Read the model definition and answer for the solid it produces. Units are mm, in the model's axes. A direction names the side the tool comes from. Give positions to 0.01 mm unless a question says otherwise; leave off trailing zeros. Loops run counter-clockwise (first coordinate to the right, second up) from the corner with the lowest first, then second, coordinate; pieces in that order, holes last. Notation, with made-up numbers: (-20, 89) -> (25, 89) arc R27 ccw to (25, 121) -> close; hole circle Ø1 at (24, 13). An arc over 180 degrees is marked (long way). One line per item, written item: value. Start each with the question number.
from build123d import *

# Parameters (mm, degrees)
SKETCH1_R           = 36
BOSS_EXTRUDE1_DEPTH = 6.35
SKETCH2_R           = 29
CUT_EXTRUDE1_DEPTH  = 52.306164347
BOSS_EXTRUDE2_START = 10
SKETCH3_R           = 45
SKETCH3_R_2         = 29
BOSS_EXTRUDE2_DEPTH = 10
CUT_EXTRUDE2_DEPTH  = 10
CUT_SWEEP1_START    = -7.7
CUT_SWEEP1_DEPTH    = 7.7
CUT_SWEEP2_START    = -7.7
CUT_SWEEP2_DEPTH    = 7.7


# Read off the part's stored shape, not the designer's step: Cut-Sweep1, Cut-Sweep2
with BuildPart() as part:
    # Sketch1 → Boss-Extrude1 (new body)
    with BuildSketch(Plane(origin=(0, 0, 0), x_dir=(1, 0, 0), z_dir=(0, 1, 0))):
        with Locations(Location((0, 0, 0), (0, 0, 270))):
            Circle(SKETCH1_R)
    extrude(amount=BOSS_EXTRUDE1_DEPTH)

    # Sketch2 → Cut-Extrude1 (cut, through all)
    with BuildSketch(Plane(origin=(0, 0, 0), x_dir=(-1, 0, 0), z_dir=(0, -1, 0))):
        with Locations(Location((0, 0, 0), (0, 0, 90))):
            Circle(SKETCH2_R)
    extrude(amount=-CUT_EXTRUDE1_DEPTH, mode=Mode.SUBTRACT)

    # Sketch3 → Boss-Extrude2 (add)
    with BuildSketch(Plane.XZ.offset(BOSS_EXTRUDE2_START)):
        with Locations(Location((0, 0, 0), (0, 0, 270))):
            Circle(SKETCH3_R)
        with Locations(Location((0, 0, 0), (0, 0, 270))):
            Circle(SKETCH3_R_2, mode=Mode.SUBTRACT)
    extrude(amount=-BOSS_EXTRUDE2_DEPTH)

    # Sketch6 → Cut-Extrude2 (cut)
    with BuildSketch(Plane(origin=(0, -10, 0), x_dir=(-1, 0, 0), z_dir=(0, -1, 0))):
        with BuildLine():
            Line((9.5, -29), (9.5, -27.399817518))
            ThreePointArc((9.5, -27.399817518), (0, -29), (-9.5, -27.399817518))
            Line((-9.5, -27.399817518), (-9.5, -29))
            Line((-9.5, -29), (-9.5, -32))
            Line((-9.5, -32), (9.5, -32))
            Line((9.5, -32), (9.5, -29))
        make_face()
        with BuildLine():
            Line((9.5, 29), (9.5, 27.399817518))
            ThreePointArc((9.5, 27.399817518), (0, 29), (-9.5, 27.399817518))
            Line((-9.5, 27.399817518), (-9.5, 29))
            Line((-9.5, 29), (-9.5, 32))
            Line((-9.5, 32), (9.5, 32))
            Line((9.5, 32), (9.5, 29))
        make_face()
    extrude(amount=-CUT_EXTRUDE2_DEPTH, mode=Mode.SUBTRACT)

    # Cut-Sweep1 outline → Cut-Sweep1 (cut)
    with BuildSketch(Plane(origin=(0, 0, 0), x_dir=(1, 0, 0), z_dir=(0, 1, 0)).offset(CUT_SWEEP1_START)):
        with BuildLine():
            add(Edge.make_bspline(
                [(9.5, 32), (13.238484468, 30.894081247), (16.809709604, 29.105075442), (23.154704566, 24.372448809), (25.850694666, 21.46020132), (27.956173262, 18.240130935)],
                knots=[0.04905898, 0.04905898, 0.04905898, 0.04905898, 0.52452949, 0.52452949, 1, 1, 1, 1], degree=3))
            Line((9.5, 32), (9.5, 27.399817518))
            ThreePointArc((9.5, 27.399817518), (18.365540323, 22.443416154), (24.978218037, 14.73392764))
            Line((24.978218037, 14.73392764), (27.956173262, 18.240130935))
        make_face()
    extrude(amount=CUT_SWEEP1_DEPTH, mode=Mode.SUBTRACT)

    # Cut-Sweep2 outline → Cut-Sweep2 (cut)
    with BuildSketch(Plane(origin=(0, 0, 0), x_dir=(1, 0, 0), z_dir=(0, 1, 0)).offset(CUT_SWEEP2_START)):
        with BuildLine():
            add(Edge.make_bspline(
                [(-9.5, -32), (-13.238484468, -30.894081248), (-16.809709604, -29.105075442), (-23.154704566, -24.372448809), (-25.850694666, -21.46020132), (-27.956173262, -18.240130935)],
                knots=[0.04905898, 0.04905898, 0.04905898, 0.04905898, 0.52452949, 0.52452949, 1, 1, 1, 1], degree=3))
            Line((-9.5, -32), (-9.5, -27.399817518))
            ThreePointArc((-9.5, -27.399817518), (-18.365540323, -22.443416154), (-24.978218037, -14.73392764))
            Line((-24.978218037, -14.73392764), (-27.956173262, -18.240130935))
        make_face()
    extrude(amount=CUT_SWEEP2_DEPTH, mode=Mode.SUBTRACT)


solid = part.part
Item 1: Section C-C, the plane y = 5 is taken. Determine the outline of the cut face in (x, z).
Item 2: Section B-B, the plane x = 0 is taken. Determine the outline of the cut face in (y, z), plus the area to 3 significant figures.
Item 3: For faces 4 (the cylindrical face through (10.81, 3.13, 34.34)), 5 (the flat face through (-11, 0, 27)), 6 (the flat face through (-9.5, -5, -30)), determine the directions among +Z, -Z, +X, -X, +Y, -Y from which every point of the face is accessible in a straight line to the end or side of a thin tool.
Item 4: Section D-D, the plane z = 34 is taken. Determine the outline of the cut face in (x, y).
Item 5: Section A-A, the plane z = 0 is taken. Determine the outline of the cut face in (x, y).
Item 6: Determine the mould class of faces 1 (the flat face through (19, -7.7, -25)), 2 (the flat face through (30.2, 0, 20.2)), 3 (the flat face through (0, -5, -32)) for opening direction Y: pulls with the +Y half, pulls with the -Y half, needs draft (parallel to the pull), parting line crosses it, or undercut.
Item 7: Flat-ended cylindrical pins translate along their axes: pin 1 (1 mm diameter, centred on x = 25.5, y = 0, fed in from +Z); pin 2 (5 mm diameter, centred on x = 4, y = -5, fed in from +Z) (3 decimals); pin 3 (1.4 mm diameter, centred on y = -3.5, z = -29.5, fed in from +X); pin 4 (5 mm diameter, centred on x = -11.5, z = 21.5, fed in from -Y). Find the tip coordinate at first contact, or state that the pin passes through.
Item 8: Consider L1, parallel to X at y = -2.25, z = 0; L2, parallel to X at y = 1, z = 0; L3, parallel to Y at x = -27, z = -24. Determine where each line is inside the solid, lowest interval first. Write a range as [from, to].
Computed values:
1. outline: circle Ø72 at (0, 0); hole circle Ø58 at (0, 0)
2. outline: (-10, -45) -> (0, -45) -> (0, -36) -> (6.35, -36) -> (6.35, -29) -> (0, -29) -> (0, -32) -> (-10, -32) -> close; (-10, 32) -> (0, 32) -> (0, 29) -> (6.35, 29) -> (6.35, 36) -> (0, 36) -> (0, 45) -> (-10, 45) -> close
2. area: 349 mm²
3. face 4: +Y
3. face 5: none
3. face 6: -Y
4. outline: (-29.48, -10) -> (29.48, -10) -> (29.48, 0) -> (11.83, 0) -> (11.83, 6.35) -> (-11.83, 6.35) -> (-11.83, 0) -> (-29.48, 0) -> close
5. outline: (-45, -10) -> (-29, -10) -> (-29, 6.35) -> (-36, 6.35) -> (-36, 0) -> (-45, 0) -> close; (29, -10) -> (45, -10) -> (45, 0) -> (36, 0) -> (36, 6.35) -> (29, 6.35) -> close
6. face 1: undercut
6. face 2: pulls with the +Y half
6. face 3: needs draft
7. pin 1: z = 37.42
7. pin 2: z = 44.975
7. pin 3: x = 34.58
7. pin 4: through
8. L1: [-45, -29], [29, 45]
8. L2: [-36, -29], [29, 36]
8. L3: [-10, 0]
